Source: three-view drawing plus pictorial views. Frame: mm from the lowest corner of the part. A direction names the side the tool comes from. Round coordinates to 2 decimals unless told otherwise and drop trailing zeros. Write each loop counter-clockwise with the first axis right and the second up, starting at its lowest first coordinate (ties: lowest second). Pieces come first, ordered by that corner, then holes. Notation, with made-up numbers: M 40,-33 L 95,-33 A8 cw 95,-21 Z; hole C -31.5,-1 d8. An arc over 180 degrees is marked long. Answer as CSV lines item,"result". Start each with the question number.
Q1. Section query A-A on y = 6. Output: boundary loops of the cut face in (x, z).
Q2. Ray query, probe 1 along Y at (x, z) = (29.25, 18.6); probe 2 along Z at (x, y) = (11.5, 6.25); probe 3 along Z at (x, y) = (3, 11.25). Return the intervals inside material, ascending.
Q3. Section query C-C on z = 19.5. Output: boundary loops of the cut face in (x, y), and give its area (3 significant figures).
Q4. Reachability of the marked faces 1, 2, 3 and 4 from +Z, -Z, +X, -X, +Y, -Y: full face, straight path, thin tool, end or side. Return the list, or none.
Q5. Section query B-B on x = 29.25. Output: boundary loops of the cut face in (y, z), and give its area (3 significant figures).
Q6. First-contact query: pin 1 (3.5 mm diameter, centred on y = 7, z = 7.5, fed in from +X); pin 2 (1 mm diameter, centred on y = 3, z = 5, fed in from -X); pin 3 (3.5 mm diameter, centred on x = 11, y = 5, fed in from +Z). Flat tips, straight axial feed; report the tip coordinate or a pass-through.
Q7. Section query D-D on x = 24. Output: boundary loops of the cut face in (y, z).
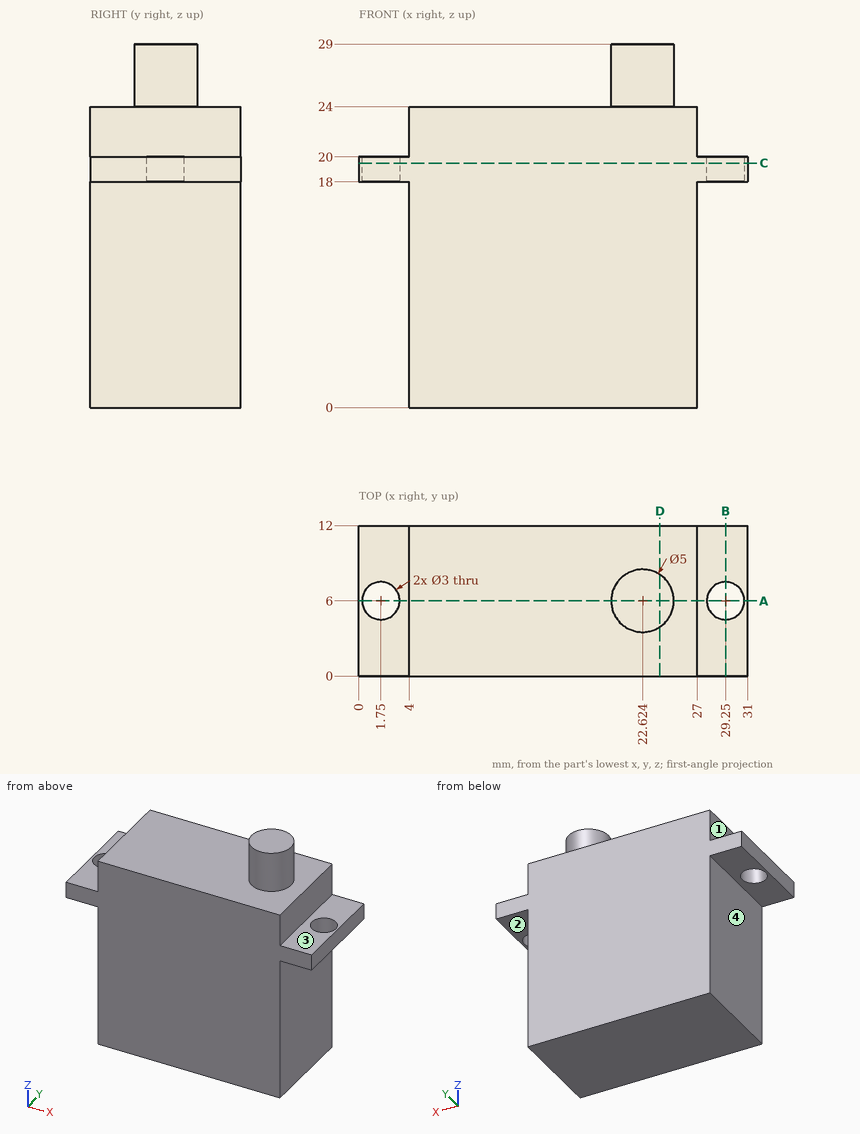
Entries:
1,outline,"M 0,18 L 0.25,18 L 0.25,20 L 0,20 Z; M 3.25,18 L 4,18 L 4,0 L 27,0 L 27,18 L 27.75,18 L 27.75,20 L 27,20 L 27,24 L 25.12,24 L 25.12,29 L 20.12,29 L 20.12,24 L 4,24 L 4,20 L 3.25,20 Z; M 30.75,18 L 31,18 L 31,20 L 30.75,20 Z"
2,probe 1,"y = 0 to 4.5, 7.5 to 12"
2,probe 2,"z = 0 to 24"
2,probe 3,"z = 18 to 20"
3,outline,"M 0,0 L 31,0 L 31,12 L 0,12 Z; hole C 1.75,6 d3; hole C 29.25,6 d3"
3,area,"358 mm^2"
4,face 1,"+Z, -X, +Y, -Y"
4,face 2,"-Z, +X, +Y, -Y"
4,face 3,"+Z, +X, +Y, -Y"
4,face 4,"-Z, -X, +Y, -Y"
5,outline,"M 0,18 L 4.5,18 L 4.5,20 L 0,20 Z; M 7.5,18 L 12,18 L 12,20 L 7.5,20 Z"
5,area,"18.0 mm^2"
6,pin 1,"stops at x = 27"
6,pin 2,"stops at x = 4"
6,pin 3,"stops at z = 24"
7,outline,"M 0,0 L 12,0 L 12,24 L 8.09,24 L 8.09,29 L 3.91,29 L 3.91,24 L 0,24 Z"
